Geometry: see drawing. Coordinates: mm, zero at the bounding-box minimum. Give positions to 0.01 mm unless a question says otherwise; leave off trailing zeros. Order: outer loops, then holes, each group sorted by start corner. A loop starts at its lowest first (then second) coordinate and runs counter-clockwise, first axis right, second up. Notation, with made-up numbers: M -37.75,51.25 L 12.25,51.25 A36 ccw 12.25,89.25 Z; hole C 1,26.5 d7. An arc over 180 degrees is marked long. Write item = value, one per line. Start each with the question number.
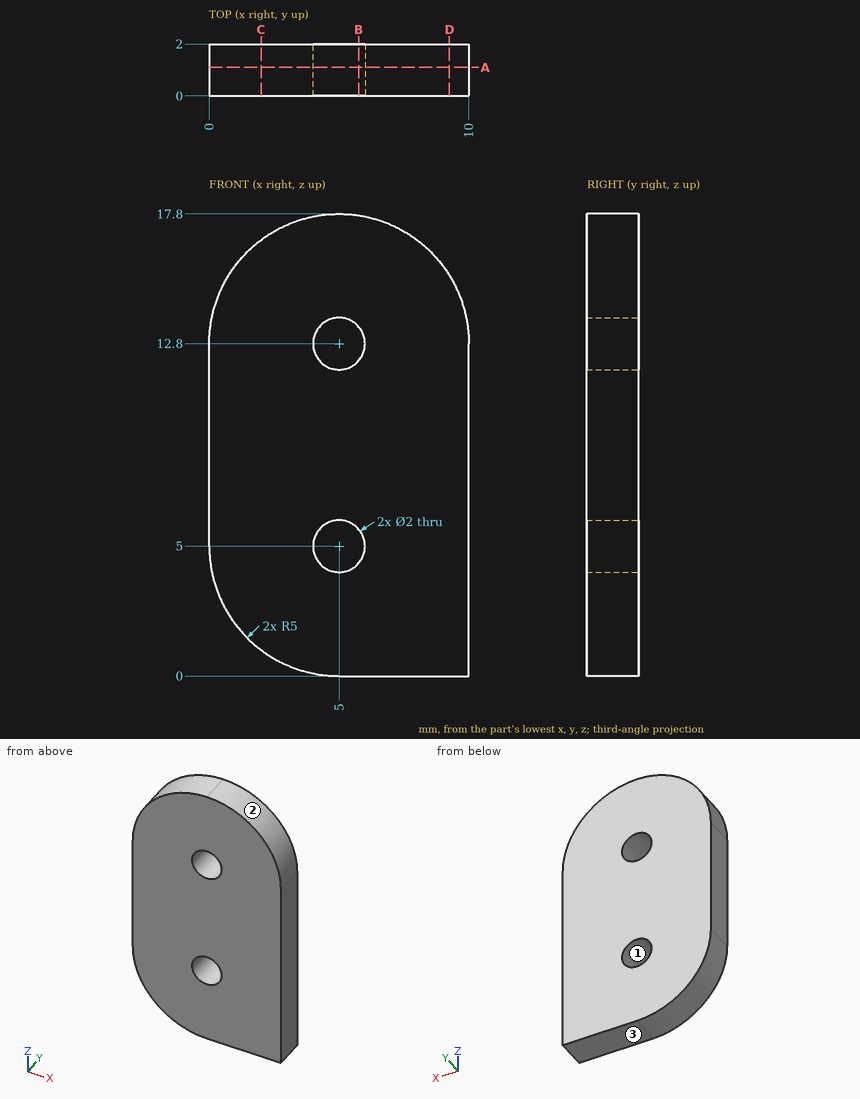
1) Ray query, L1, parallel to Z at x = 5, y = 0.8; L2, parallel to Z at x = 4.5, y = 0.55; L3, parallel to X at y = 0.85, z = 4.75. Return the intervals inside material, ascending.
2) Cut plane A-A (y = 1.1). Give the number of separate pieces and of enclosed holes in the cut face, plus the area to 3 significant figures.
3) Cut plane C-C (x = 2). Return loops of the section in (y, z).
4) Cut plane B-B (x = 5.75). Return loops of the section in (y, z), plus the area to 3 significant figures.
5) Cut plane D-D (x = 9.25). Return loops of the section in (y, z).
6) Draft query along X for the marked faces 1, 2 and 3. Return one class per face: pulls with the +X half, pulls with the -X half, needs draft (parallel to the pull), parting line crosses it, or undercut.
Reply:
q1.L1 = 0 to 4, 6 to 11.8, 13.8 to 17.8
q1.L2 = 0.03 to 4.13, 5.87 to 11.93, 13.67 to 17.77
q1.L3 = 0.01 to 4.03, 5.97 to 10
q2.separate_pieces = 1
q2.enclosed_holes = 2
q2.area = 156 mm²
q3.outline = M 0,1 L 2,1 L 2,16.8 L 0,16.8 Z
q4.outline = M 0,0 L 2,0 L 2,4.34 L 0,4.34 Z; M 0,5.66 L 2,5.66 L 2,12.14 L 0,12.14 Z; M 0,13.46 L 2,13.46 L 2,17.74 L 0,17.74 Z
q4.area = 30.2 mm²
q5.outline = M 0,0 L 2,0 L 2,15.43 L 0,15.43 Z
q6.face_1 = undercut
q6.face_2 = pulls with the +X half
q6.face_3 = needs draft
